Could you check a few things on this drawing? It's one solid part, dimensions in mm from its lowest x, y, z. A direction names the side the tool comes from. Round coordinates to 2 decimals unless told otherwise and drop trailing zeros. Loops run counter-clockwise (first coordinate to the right, second up) from the corner with the lowest first, then second, coordinate; pieces in that order, holes last. Notation, with made-up numbers: M -16.5,48.25 L 38.5,48.25 A9 ccw 38.5,61.25 Z; hole C 54.25,6 d10. An arc over 180 degrees is marked long. Answer as a JSON object with one key per item and string values.
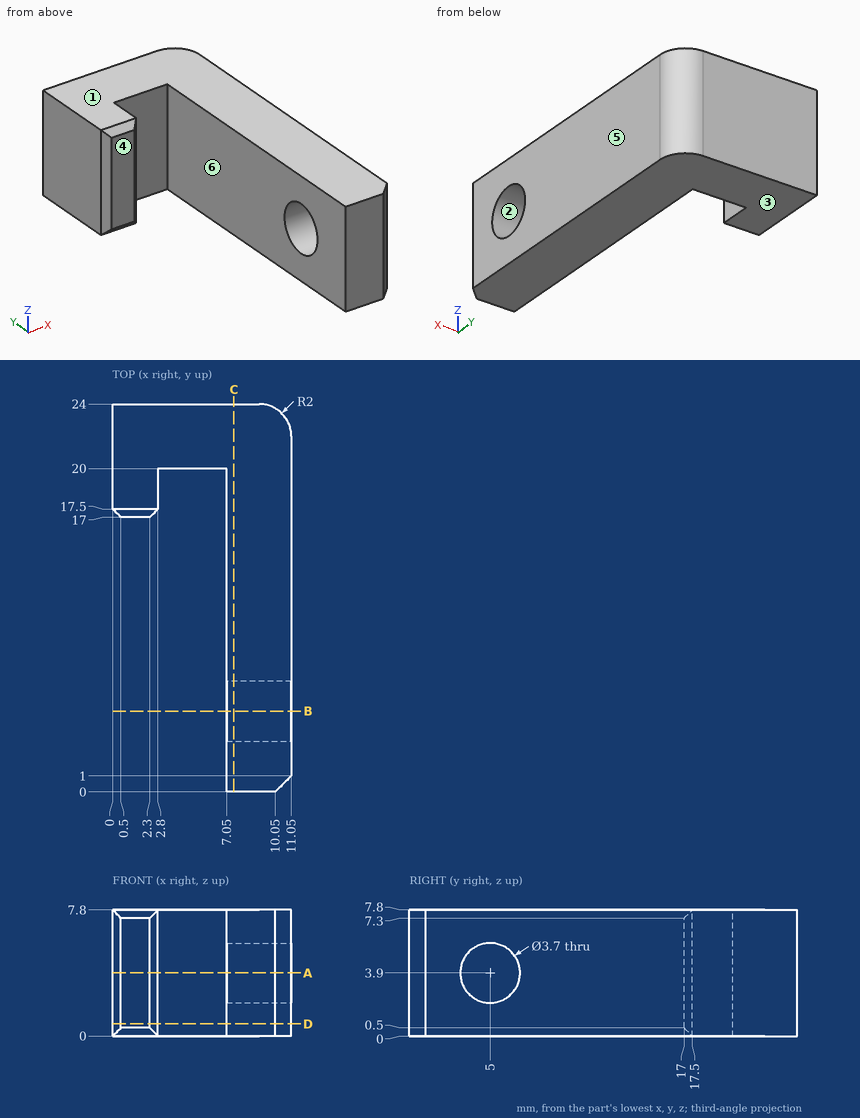
Item 1: If we mould it in two halves opening along Z, with no side actions, what happens to the marked faces 1, 2 and 3? For each: pulls with the +Z half, pulls with the -Z half, needs draft (parallel to the pull), parting line crosses it, or undercut.
Resolved:
{"face 1": "pulls with the +Z half", "face 2": "undercut", "face 3": "pulls with the -Z half"}
Item 2: I'm going to push flat-ended pins straight in: pin 1 Ø4 at (y, z) = (9.5, 5.5) entering from -X; pin 2 Ø0.9 at (x, z) = (1.5, 4.5) entering from -Y. Where does each tip first touch, or does it pass through?
Resolved:
{"pin 1": "x = 7.05", "pin 2": "y = 17"}
Item 3: Please list where these lines run through material, in increasing order: probe 1 along Z at (x, y) = (8.8, 5); probe 2 along X at (y, z) = (10.75, 1.25); probe 3 along Y at (x, z) = (4, 3). Write a range as from..to.
Resolved:
{"probe 1": "0..2.05, 5.75..7.8", "probe 2": "7.05..11.05", "probe 3": "20..24"}
Item 4: On a 3-axis mill with a long thin cutter (end or side, diameter ignored), from which of +Z, -Z, +X, -X, +Y, -Y can I reach the whole of each face in a straight line? I mean the marked faces 4, 5 and 6. Say none if no direction works.
Resolved:
{"face 4": "+Z, -Z, -X, -Y", "face 5": "+Z, -Z, +X, +Y, -Y", "face 6": "+Z, -Z, -Y"}
Item 5: I want a section at C-C, the plane x = 7.5. Please give me the cut outline in (y, z).
Resolved:
{"outline": "M 0,0 L 24,0 L 24,7.8 L 0,7.8 Z; hole C 5,3.9 d3.7"}
Item 6: I want a section at D-D, the plane z = 0.75. Please give me the cut outline in (x, y).
Resolved:
{"outline": "M 0,17.5 L 0.5,17 L 2.3,17 L 2.8,17.5 L 2.8,20 L 7.05,20 L 7.05,0 L 10.05,0 L 11.05,1 L 11.05,22 A2 ccw 9.05,24 L 0,24 Z"}
Item 7: I want a section at B-B, the plane y = 5. Please give me the cut outline in (x, z).
Resolved:
{"outline": "M 7.05,0 L 11.05,0 L 11.05,2.05 L 7.05,2.05 Z; M 7.05,5.75 L 11.05,5.75 L 11.05,7.8 L 7.05,7.8 Z"}
Item 8: I want a section at A-A, the plane z = 3.9. Please give me the cut outline in (x, y).
Resolved:
{"outline": "M 0,17.5 L 0.5,17 L 2.3,17 L 2.8,17.5 L 2.8,20 L 7.05,20 L 7.05,6.85 L 11.05,6.85 L 11.05,22 A2 ccw 9.05,24 L 0,24 Z; M 7.05,0 L 10.05,0 L 11.05,1 L 11.05,3.15 L 7.05,3.15 Z"}
